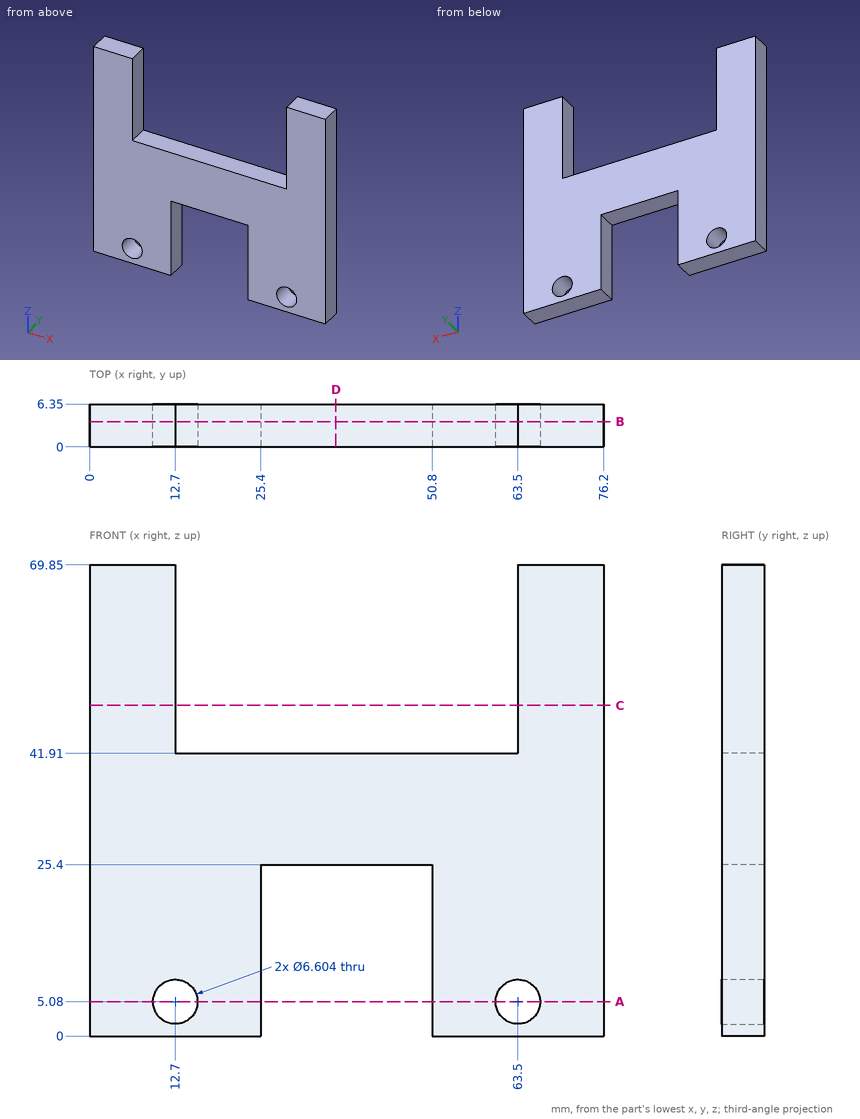
Input: dimensioned drawing with shaded views. Units: mm. Origin: part minimum x, y, z. Coordinates: 2 decimals unless noted, no trailing zeros. Order: outer loops, then holes, each group sorted by start corner. A loop starts at its lowest first (then second) coordinate and runs counter-clockwise, first axis right, second up.
1. Cut plane A-A, the plane z = 5.08. Return loops of the section in (x, y).
Checked values:
outline: (0, 0) - (9.4, 0) - (9.4, 6.35) - (0, 6.35) - close; (16, 0) - (25.4, 0) - (25.4, 6.35) - (16, 6.35) - close; (50.8, 0) - (60.2, 0) - (60.2, 6.35) - (50.8, 6.35) - close; (66.8, 0) - (76.2, 0) - (76.2, 6.35) - (66.8, 6.35) - close
2. Ray query, line 1 along X through (y, z) = (4.25, 5.08); line 2 along X through (y, z) = (0.75, 44); line 3 along X through (y, z) = (0.75, 19.5). Return the intervals inside material, ascending.
Checked values:
line 1: x = 0 to 9.4, 16 to 25.4, 50.8 to 60.2, 66.8 to 76.2
line 2: x = 0 to 12.7, 63.5 to 76.2
line 3: x = 0 to 25.4, 50.8 to 76.2
3. Contact query for flat-ended pins moving along their axis: P1, Ø2, axis at x = 49, y = 3, coming from the -Z side; P2, Ø1, axis at x = 34, y = 2.5, coming from the +Z side. Output: stop coordinate, or through.
Checked values:
P1: stops at z = 25.4
P2: stops at z = 41.91
4. Cut plane D-D, the plane x = 36.5. Return loops of the section in (y, z), plus the area to 3 significant figures.
Checked values:
outline: (0, 25.4) - (6.35, 25.4) - (6.35, 41.91) - (0, 41.91) - close
area: 105 mm2
5. Cut plane B-B, the plane y = 3.75. Return loops of the section in (x, z), plus the area to 3 significant figures.
Checked values:
outline: (0, 0) - (25.4, 0) - (25.4, 25.4) - (50.8, 25.4) - (50.8, 0) - (76.2, 0) - (76.2, 69.85) - (63.5, 69.85) - (63.5, 41.91) - (12.7, 41.91) - (12.7, 69.85) - (0, 69.85) - close; hole circle Ø6.6 at (12.7, 5.08); hole circle Ø6.6 at (63.5, 5.08)
area: 3,190 mm2
6. Cut plane C-C, the plane z = 49. Return loops of the section in (x, y).
Checked values:
outline: (0, 0) - (12.7, 0) - (12.7, 6.35) - (0, 6.35) - close; (63.5, 0) - (76.2, 0) - (76.2, 6.35) - (63.5, 6.35) - close
